Could you check a few things on this model? Use its own coordinates, in mm. Give positions to 0.01 mm unless a question says otherwise; leave off trailing zeros. Loops run counter-clockwise (first coordinate to the right, second up) from the corner with the lowest first, then second, coordinate; pieces in that order, holes last. Notation, with made-up numbers: (14, -19) -> (50, -19) arc R27 ccw to (50, 16) -> close; hole circle Ø4 at (51, -32). An arc over 180 degrees is marked (long way). Write item = value, one per line. Start each with the question number.
1) I need wall thicknesses on probe 1 along Y at (x, z) = (9.25, 1.55); probe 2 along Y at (x, z) = (0.5, 1.1); probe 3 along X at (y, z) = (-2, 1.4). Which ranges of each line are inside material? Lowest first, please. Write a range as from..to.
2) I want a section at A-A (x = 0). List the corners of the cut face in (y, z) for me, and give its area (3 significant figures).
3) I'm going to push a flat-ended pin straight in: pin 1 Ø0.6 at (y, z) = (3.5, 1.5) entering from -X. Where does the tip first touch, or does it pass through?
4) If we mould it in two halves opening along X, with no side actions, what happens to faces 1 (the face through (9.56, 4.33, 1.58)), 2 (the face through (9.56, 4.98, 0.59)), 3 (the face through (-8.822, -6.764, 1.681)), 4 (the face through (0, 0, 2))? For each: +X half, -X half, draft (parallel to the pull), parting line (faces both ways), or undercut.
from build123d import *

# Parameters (mm, degrees)
SKETCH1_R           = 11.9
SKETCH1_W           = 2.4
SKETCH1_H           = 5
BOSS_EXTRUDE2_DEPTH = 2
BOSS_EXTRUDE2_TAPER = 25
SKETCH4_W           = 1.199715213
SKETCH4_H           = 2.206755838
CUT_EXTRUDE1_DEPTH  = 2


with BuildPart() as part:
    # Sketch1 → Boss-Extrude2 (new body)
    with BuildSketch(Plane.XY):
        Circle(SKETCH1_R)
        with Locations((10, 0)):
            Rectangle(SKETCH1_W, SKETCH1_H, mode=Mode.SUBTRACT)
    extrude(amount=BOSS_EXTRUDE2_DEPTH, taper=BOSS_EXTRUDE2_TAPER)

    # Sketch4 → Cut-Extrude1 (cut)
    with BuildSketch(Plane(origin=(0, 2.053484512, -0.957555554), x_dir=(1, 0, 0), z_dir=(0, -0.9063077870366496, 0.42261826174070033))):
        with Locations((9.570937649, 2.159923573)):
            Rectangle(SKETCH4_W, SKETCH4_H)
    extrude(amount=-CUT_EXTRUDE1_DEPTH, mode=Mode.SUBTRACT)


solid = part.part
Answer list:
q1.probe_1 = -6.27..-3.22, 4.4..6.27
q1.probe_2 = -11.38..11.38
q1.probe_3 = -11.07..8.15
q2.outline = (-11.9, 0) -> (11.9, 0) -> (10.97, 2) -> (-10.97, 2) -> close
q2.area = 45.7 mm^2
q3.pin_1 = -10.81
q4.face_1 = undercut
q4.face_2 = undercut
q4.face_3 = parting line
q4.face_4 = draft
